Geometry: see drawing. Coordinates: mm, zero at the bounding-box minimum. A direction names the side the tool comes from. Round coordinates to 2 decimals unless told otherwise and drop trailing zeros. Loops run counter-clockwise (first coordinate to the right, second up) from the corner with the lowest first, then second, coordinate; pieces in that order, holes last. Notation, with made-up numbers: (42.25, 64.25) - (66.25, 64.25) arc R27 cw to (66.25, 87.25) - close; hole circle Ø1 at (87.5, 60). An arc over 180 degrees is marked (long way). Write item = value, one per line. Start each with the question number.
Item 1: First-contact query: pin 1 (5 mm diameter, centred on x = 7, z = 9.5, fed in from +Y); pin 2 (2.5 mm diameter, centred on y = 5, z = 4.5, fed in from -X). Flat tips, straight axial feed; report the tip coordinate or a pass-through.
Item 2: Section C-C (z = 7.3). Return loops of the section in (x, y), plus the area to 3 significant figures.
Item 3: Line query: line 1 (Z direction, x = 20.25, y = 3.4); line 2 (X direction, y = 4.05, z = 7.75); line 3 (X direction, y = 2.05, z = 7.3). Output: solid intervals per line, ascending. Write a range as from..to.
Item 4: Section A-A (x = 4.2). Return loops of the section in (y, z), plus the area to 3 significant figures.
Item 5: Draft query along Z for the marked faces 4, 5 and 6. Return one class per face: pulls with the +Z half, pulls with the -Z half, needs draft (parallel to the pull), parting line crosses it, or undercut.
Item 6: Section B-B (y = 3.25). Return loops of the section in (x, z).
Item 7: Section D-D (x = 8.75). Return loops of the section in (y, z), plus the area to 3 significant figures.
Item 8: Access query for the marked faces 1, 2 and 3. Directions: +Z, -Z, +X, -X, +Y, -Y. A direction counts if a zero-diameter tool reaches every point of the face in a straight line with its end or side. Return the directions, or none.
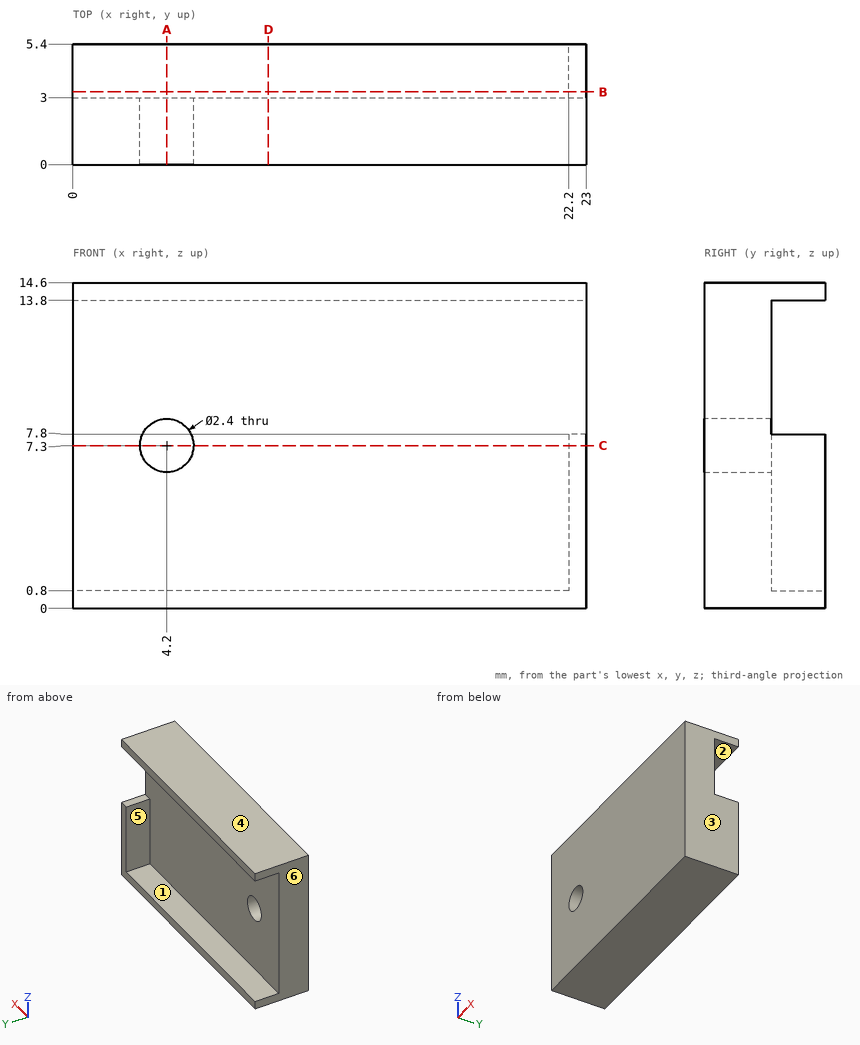
Taken from the geometry:
q1.pin_1 = 3
q1.pin_2 = 22.2
q2.outline = (0, 0) - (3, 0) - (3, 3) - (0, 3) - close; (5.4, 0) - (23, 0) - (23, 5.4) - (22.2, 5.4) - (22.2, 3) - (5.4, 3) - close
q2.area = 63.7 mm^2
q3.line_1 = 0..0.8, 13.8..14.6
q3.line_2 = 22.2..23
q3.line_3 = 0..3, 5.4..23
q4.outline = (0, 0) - (5.4, 0) - (5.4, 0.8) - (3, 0.8) - (3, 6.1) - (0, 6.1) - close; (0, 8.5) - (3, 8.5) - (3, 13.8) - (5.4, 13.8) - (5.4, 14.6) - (0, 14.6) - close
q4.area = 40.4 mm^2
q5.face_4 = pulls with the +Z half
q5.face_5 = undercut
q5.face_6 = needs draft
q6.outline = (0, 0) - (23, 0) - (23, 7.8) - (22.2, 7.8) - (22.2, 0.8) - (0, 0.8) - close; (0, 13.8) - (23, 13.8) - (23, 14.6) - (0, 14.6) - close
q7.outline = (0, 0) - (5.4, 0) - (5.4, 0.8) - (3, 0.8) - (3, 13.8) - (5.4, 13.8) - (5.4, 14.6) - (0, 14.6) - close
q7.area = 47.6 mm^2
q8.face_1 = -X, +Y
q8.face_2 = +X, -X, +Y
q8.face_3 = +Z, -Z, +X, +Y, -Y
